from build123d import *

# Parameters (mm, degrees)
SALIENTE_EXTRUIR1_DEPTH                              = 10
SALIENTE_EXTRUIR2_DEPTH                              = 10
CROQUIS3_R                                           = 26.5
CORTAR_EXTRUIR1_DEPTH                                = 10
REFRENTADO_PARA_TORNILLO_CON_CABEZA_HUEC_D           = 6.6
REFRENTADO_PARA_TORNILLO_CON_CABEZA_HUEC_CBORE_D     = 11
REFRENTADO_PARA_TORNILLO_CON_CABEZA_HUEC_CBORE_DEPTH = 4.4


with BuildPart() as part:
    # Croquis1 → Saliente-Extruir1 (new body)
    with BuildSketch(Plane(origin=(0, 0, 0), x_dir=(1, 0, 0), z_dir=(0, 1, 0))):
        with BuildLine():
            Line((-70, -70), (-70, 70))
            ThreePointArc((-70, 70), (-52.983030462, 76.249658661), (-44.055908755, 92.027554074))
            ThreePointArc((-44.055908755, 92.027554074), (-36.156795126, 78.313355526), (-21.147629234, 83.333333333))
            ThreePointArc((-21.147629234, 83.333333333), (0, 95), (21.147629234, 83.333333333))
            ThreePointArc((21.147629234, 83.333333333), (36.156795126, 78.313355526), (44.055908755, 92.027554074))
            ThreePointArc((44.055908755, 92.027554074), (52.983030462, 76.249658661), (70, 70))
            Line((70, 70), (70, -70))
            ThreePointArc((70, -70), (52.983030462, -76.249658661), (44.055908755, -92.027554074))
            ThreePointArc((44.055908755, -92.027554074), (36.156795126, -78.313355526), (21.147629234, -83.333333333))
            ThreePointArc((21.147629234, -83.333333333), (0, -95), (-21.147629234, -83.333333333))
            ThreePointArc((-21.147629234, -83.333333333), (-36.156795126, -78.313355526), (-44.055908755, -92.027554074))
            ThreePointArc((-44.055908755, -92.027554074), (-52.983030462, -76.249658661), (-70, -70))
        make_face()
    extrude(amount=SALIENTE_EXTRUIR1_DEPTH)

    # Croquis2 → Saliente-Extruir2 (add)
    with BuildSketch(Plane(origin=(0, 10, 0), x_dir=(1, 0, 0), z_dir=(0, 1, 0))):
        with BuildLine():
            Line((-70, 25.98076189), (-70, 70))
            ThreePointArc((-70, 70), (-85.909969357, 57.627811916), (-77.837993487, 39.160506523))
            ThreePointArc((-77.837993487, 39.160506523), (-72.107558403, 33.647896498), (-70, 25.98076189))
        make_face()
        with BuildLine():
            ThreePointArc((77.837993487, 39.160506523), (85.909969357, 57.627811916), (70, 70))
            Line((70, 70), (70, 25.98076213))
            ThreePointArc((70, 25.98076213), (72.107558465, 33.647896602), (77.837993487, 39.160506523))
        make_face()
        with BuildLine():
            ThreePointArc((77.5, 12.990381057), (72.009618939, 18.480762121), (70, 25.98076213))
            Line((70, 25.98076213), (70, -25.98076213))
            ThreePointArc((70, -25.98076213), (72.009618939, -18.480762121), (77.5, -12.990381057))
            ThreePointArc((77.5, -12.990381057), (85, 0), (77.5, 12.990381057))
        make_face()
        with BuildLine():
            Line((-70, -25.980762199), (-70, 25.98076189))
            ThreePointArc((-70, 25.98076189), (-72.009618999, 18.480762017), (-77.5, 12.990381057))
            ThreePointArc((-77.5, 12.990381057), (-85, 0), (-77.5, -12.990381057))
            ThreePointArc((-77.5, -12.990381057), (-72.009618922, -18.480762151), (-70, -25.980762199))
        make_face()
        with BuildLine():
            Line((-70, -70), (-70, -25.980762199))
            ThreePointArc((-70, -25.980762199), (-72.107558482, -33.647896631), (-77.837993487, -39.160506523))
            ThreePointArc((-77.837993487, -39.160506523), (-85.909969357, -57.627811916), (-70, -70))
        make_face()
        with BuildLine():
            ThreePointArc((77.837993487, -39.160506523), (72.107558465, -33.647896602), (70, -25.98076213))
            Line((70, -25.98076213), (70, -70))
            ThreePointArc((70, -70), (85.909969357, -57.627811916), (77.837993487, -39.160506523))
        make_face()
    extrude(amount=-SALIENTE_EXTRUIR2_DEPTH)

    # Croquis3 → Cortar-Extruir1 (cut)
    with BuildSketch(Plane(origin=(0, 10, 0), x_dir=(1, 0, 0), z_dir=(0, 1, 0))):
        with Locations(Location((0, 0, 0), (0, 0, 270))):
            Circle(CROQUIS3_R)
    extrude(amount=-CORTAR_EXTRUIR1_DEPTH, mode=Mode.SUBTRACT)

    # Refrentado para tornillo con cabeza hueca de M61 (through all)
    with Locations(Plane(origin=(-55, 0, 57.5), x_dir=(0, 0, -1), z_dir=(0, -1, 0))):
        with Locations((0, 0), (0, 110), (115, 110), (115, 0), (57.5, 55)):
            CounterBoreHole(REFRENTADO_PARA_TORNILLO_CON_CABEZA_HUEC_D / 2, REFRENTADO_PARA_TORNILLO_CON_CABEZA_HUEC_CBORE_D / 2, REFRENTADO_PARA_TORNILLO_CON_CABEZA_HUEC_CBORE_DEPTH)


solid = part.part
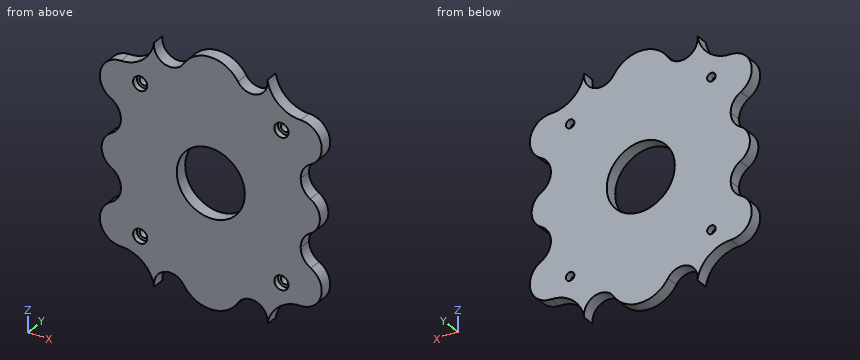
Geometry check sheet. Reference: the model listing, model coordinates, mm. Give positions to 0.01 mm unless a question says otherwise; leave off trailing zeros. Write each loop counter-clockwise with the first axis right and the second up, starting at its lowest first coordinate (ties: lowest second). Pieces come first, ordered by that corner, then holes.
1) Thickness scan on line 1 (X direction, y = 1.15, z = -57.5); line 2 (X direction, y = 7.3, z = 57.5); line 3 (Z direction, x = -74, y = 9.5). Record the ranges inside material, lowest first.
Values follow:
line 1: x = -85.94 to -60.5, -49.5 to 49.5, 60.5 to 85.94
line 2: x = -85.94 to -58.3, -51.7 to 51.7, 58.3 to 85.94
line 3: z = -69.51 to -36.18, -15.78 to 15.78, 36.18 to 69.51
2) Cross-section at A-A (y = 2). Record the boundary of the cut face in (x, z).
Values follow:
outline: (-77.84, -39.16) arc R16.42 ccw to (-70, -70) arc R26.29 cw to (-44.06, -92.03) arc R12.5 cw to (-21.15, -83.33) arc R25 ccw to (21.15, -83.33) arc R12.5 cw to (44.06, -92.03) arc R26.29 cw to (70, -70) arc R16.42 ccw to (77.84, -39.16) arc R15 cw to (77.5, -12.99) arc R15 ccw to (77.5, 12.99) arc R15 cw to (77.84, 39.16) arc R16.42 ccw to (70, 70) arc R26.29 cw to (44.06, 92.03) arc R12.5 cw to (21.15, 83.33) arc R25 ccw to (-21.15, 83.33) arc R12.5 cw to (-44.06, 92.03) arc R26.29 cw to (-70, 70) arc R16.42 ccw to (-77.84, 39.16) arc R15 cw to (-77.5, 12.99) arc R15 ccw to (-77.5, -12.99) arc R15 cw to start; hole circle Ø11 at (-55, -57.5); hole circle Ø11 at (-55, 57.5); hole circle Ø53 at (0, 0); hole circle Ø11 at (55, -57.5); hole circle Ø11 at (55, 57.5)
3) Cross-section at D-D (x = 0). Record the boundary of the cut face in (y, z).
Values follow:
outline: (0, -95) - (10, -95) - (10, -26.5) - (0, -26.5) - close; (0, 26.5) - (10, 26.5) - (10, 95) - (0, 95) - close
4) Cross-section at B-B (x = -74). Record the boundary of the cut face in (y, z), plus the area to 3 significant figures.
Values follow:
outline: (0, -69.51) - (10, -69.51) - (10, -36.18) - (0, -36.18) - close; (0, -15.78) - (10, -15.78) - (10, 15.78) - (0, 15.78) - close; (0, 36.18) - (10, 36.18) - (10, 69.51) - (0, 69.51) - close
area: 982 mm2
5) Cross-section at C-C (z = 57.5). Record the boundary of the cut face in (x, y).
Values follow:
outline: (-85.94, 0) - (-60.5, 0) - (-60.5, 4.4) - (-58.3, 4.4) - (-58.3, 10) - (-85.94, 10) - close; (-51.7, 4.4) - (-49.5, 4.4) - (-49.5, 0) - (49.5, 0) - (49.5, 4.4) - (51.7, 4.4) - (51.7, 10) - (-51.7, 10) - close; (58.3, 4.4) - (60.5, 4.4) - (60.5, 0) - (85.94, 0) - (85.94, 10) - (58.3, 10) - close
6) Go/stop test with flat-tipped pins: pin 1 Ø8.5 at (x, z) = (55, 57.5) entering from -Y; pin 2 Ø1.5 at (x, y) = (-61.5, 1.5) entering from -Z; pin 3 Ø5.5 at (x, z) = (-55, -57.5) entering from -Y; pin 4 Ø1 at (y, z) = (2, 54.5) entering from -X. Record where each tip stops, or that it passes through.
Values follow:
pin 1: stops at y = 4.4
pin 2: stops at z = -71.68
pin 3: passes through
pin 4: stops at x = -86.41
